CAD build for the part. Positions are in the model's coordinates, mm. Face numbers are marked on the shaded views. A direction names the side the tool comes from. Round coordinates to 2 decimals unless told otherwise and drop trailing zeros. Order: outer loops, then holes, each group sorted by start corner. A loop starts at its lowest first (then second) coordinate and runs counter-clockwise, first axis right, second up. Notation, with made-up numbers: (59, 88.5) -> (113, 88.5) arc R19 ccw to (113, 99.5) -> close; hole circle Ø4 at (-35, 38.25). An arc over 180 degrees is marked (long way). Return JSON: item names as keys, results as strings. Group by question number.
Q1. Probe line 1 along Y through (x, z) = (0, 2.5); line 2 along X through (y, z) = (-4, 1.5); line 3 along Y through (x, z) = (-6.5, 1.5). List the from-to ranges inside material, lowest first.
Q2. Cut at A-A (x = 0). Write the cut outline in (y, z), then the cut area to 3 significant figures.
Q3. Cut at C-C (z = 8). Write the cut outline in (x, y).
Q4. Mould opens along X. For the marked faces 3, 4 and 5 say: +X half, -X half, draft (parallel to the pull), parting line (faces both ways), or undercut.
Q5. Cut at B-B (y = 0). Write the cut outline in (x, z), then the cut area to 3 significant figures.
Q6. Flat gauge pins, fed straight in: pin 1 (4 mm diameter, centred on x = 6.93, y = -4, fed in from +Z); pin 2 (8 mm diameter, centred on x = -7, z = 5.5, fed in from -Y); pin 3 (8 mm diameter, centred on x = -4.5, z = 13.5, fed in from +Y). Where does each tip first touch, or does it go through?
Q7. Which spindle directions (+Z, -Z, +X, -X, +Y, -Y) get a long thin tool onto all of the face, cutting with end or side? Do the marked faces 1 and 2. Say none if no direction does.
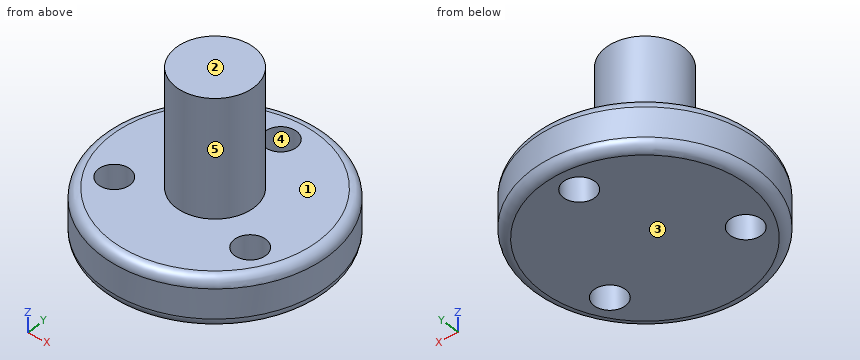
Autodesk Inventor part; units mm, degrees
ref_plane "YZ Plane" through (0, 0, 0) normal (1, 0, 0) x (0, 1, 0)
ref_plane "XZ Plane" through (0, 0, 0) normal (0, 1, 0) x (-1, 0, 0)
ref_plane "XY Plane" through (0, 0, 0) normal (0, 0, 1) x (1, 0, 0)
sketch "Sketch1" plane through (0, 0, 0) normal (0, 0, 1) x (1, 0, 0)
  circle A0 centre (0, 0) radius 11.5
  dimension "d0" = 23
extrude "Extrusion1" add sketch "Sketch1" along normal blind 5
sketch "Sketch2" plane through (0, 0, 5) normal (0, 0, 1) x (1, 0, 0)
  circle A0 centre (0, 0) radius 3.95
  dimension "d3" = 7.9
extrude "Extrusion2" add sketch "Sketch2" along normal blind 12
sketch "Sketch3" plane through (0, 0, 0) normal (0, 0, -1) x (-1, 0, 0)
  circle A0 centre (0, 0) radius 4
  point P0 (0, 8)
  point P1 (-6.9282, -4)
  point P2 (6.9282, -4)
  dimension "d8" = 360
  dimension "d17" = 8
hole "Hole1" at (0, 8, 0) at (6.9282, -4, 0) at (-6.9282, -4, 0) direction (0, 0, 1) diameter 3.2 end through all
fillet "Fillet1" radius 1 2 edges at (-11.5, 0, 0) (-11.5, 0, 5)
properties part number "Eixo de suporte II"
Solution:
{
 "1": {"line 1": "y = -11.5 to 6.4, 9.6 to 11.5", "line 2": "x = -10.78 to -8.53, -5.33 to 5.33, 8.53 to 10.78", "line 3": "y = -9.49 to -5.54, -2.46 to 9.49"},
 "2": {"outline": "(-11.5, 1) arc R1 ccw to (-10.5, 0) -> (6.4, 0) -> (6.4, 5) -> (3.95, 5) -> (3.95, 17) -> (-3.95, 17) -> (-3.95, 5) -> (-10.5, 5) arc R1 ccw to (-11.5, 4) -> close; (9.6, 0) -> (10.5, 0) arc R1 ccw to (11.5, 1) -> (11.5, 4) arc R1 ccw to (10.5, 5) -> (9.6, 5) -> close", "area": "193 mm²"},
 "3": {"outline": "circle Ø7.9 at (0, 0)"},
 "4": {"face 3": "draft", "face 4": "undercut", "face 5": "parting line"},
 "5": {"outline": "(-11.5, 1) arc R1 ccw to (-10.5, 0) -> (10.5, 0) arc R1 ccw to (11.5, 1) -> (11.5, 4) arc R1 ccw to (10.5, 5) -> (3.95, 5) -> (3.95, 17) -> (-3.95, 17) -> (-3.95, 5) -> (-10.5, 5) arc R1 ccw to (-11.5, 4) -> close", "area": "209 mm²"},
 "6": {"pin 1": "stops at z = 5", "pin 2": "stops at y = -11.03", "pin 3": "stops at y = 3.92"},
 "7": {"face 1": "+Z", "face 2": "+Z, +X, -X, +Y, -Y"}
}
